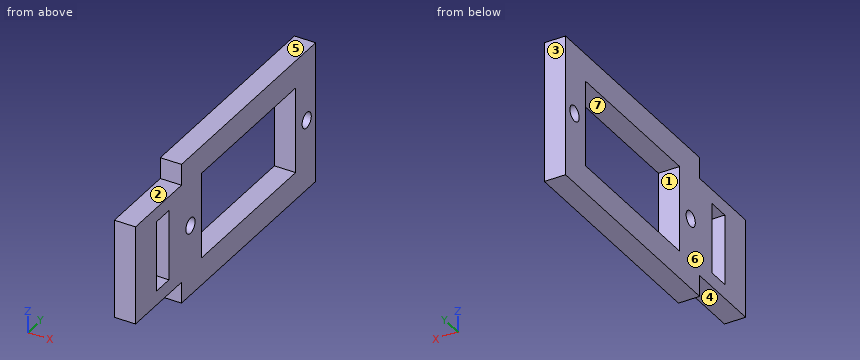
```python
from build123d import *

# Parameters (mm, degrees)
SKETCH1_W           = 20
SKETCH1_H           = 43.1
SKETCH1_W_2         = 10
SKETCH1_H_2         = 3
BOSS_EXTRUDE1_DEPTH = 3
SKETCH2_R           = 1.1
SKETCH2_W           = 12.2
SKETCH2_H           = 22.5
SKETCH2_W_2         = 3
SKETCH2_H_2         = 11
CUT_EXTRUDE1_DEPTH  = 3


with BuildPart() as part:
    # Sketch1 → Boss-Extrude1 (new body)
    with BuildSketch(Plane(origin=(0, 0, 0), x_dir=(0, 0, -1), z_dir=(1, 0, 0))):
        with Locations((10, 21.55)):
            Rectangle(SKETCH1_W, SKETCH1_H)
        with Locations((10, 6.5)):
            Rectangle(SKETCH1_W_2, SKETCH1_H_2, mode=Mode.SUBTRACT)
    extrude(amount=BOSS_EXTRUDE1_DEPTH)

    # Sketch2 → Cut-Extrude1 (cut)
    with BuildSketch(Plane.ZY):
        with Locations((-10, 40.95)):
            Circle(SKETCH2_R)
        with Locations((-10, 13.15)):
            Circle(SKETCH2_R)
        with Locations((-10, 27.05)):
            Rectangle(SKETCH2_W, SKETCH2_H)
        with Locations((-18.5, 5.5)):
            Rectangle(SKETCH2_W_2, SKETCH2_H_2)
        with Locations((-1.5, 5.5)):
            Rectangle(SKETCH2_W_2, SKETCH2_H_2)
    extrude(amount=-CUT_EXTRUDE1_DEPTH, mode=Mode.SUBTRACT)


solid = part.part
```
Model file for the job. Use its own axes, mm. Face numbers are marked on the shaded views. A direction names the side the tool comes from. Coordinates: 2 decimals unless noted, no trailing zeros. Write each loop counter-clockwise with the first axis right and the second up, starting at its lowest first coordinate (ties: lowest second). Pieces come first, ordered by that corner, then holes. Notation, with made-up numbers: (0, 69) - (32, 69) arc R25 ccw to (32, 96) - close; hole circle Ø1 at (-27.75, 89.25). An arc over 180 degrees is marked (long way). One line per item, written item: value. Start each with the question number.
1. Slice it at C-C (y = 13.15). Write the cut outline in (x, z).
2. Slice it at D-D (z = -12.75). Write the cut outline in (x, y), plus the area to 3 significant figures.
3. Probe line 1 (Y direction, x = 2.2, z = -10); line 2 (Y direction, x = 0.8, z = -14); line 3 (Z direction, x = 0.7, y = 30). List the from-to ranges inside material, lowest first. Write a range as from..to.
4. Mould opens along Z. For the marked faces 5, 6 and 7 say: released by +Z, released by -Z, zero draft, split by the parting line, or undercut.
5. Slice it at A-A (z = -10). Write the cut outline in (x, y).
6. Flat gauge pins, fed straight in: pin 1 (5 mm diameter, centred on y = 11, z = -12.5, fed in from -X); pin 2 (1.5 mm diameter, centred on x = 1.5, y = 7, fed in from -Z); pin 3 (1.3 mm diameter, centred on y = 13.15, z = -10, fed in from -X); pin 4 (1.5 mm diameter, centred on x = 2, y = 7, fed in from +Z). Where does each tip first touch, or does it go through?
7. Slice it at B-B (x = 1.4). Write the cut outline in (y, z).
8. Tool access for the marked faces 1, 2, 3 and 4: list every direction of +Z, -Z, +X, -X, +Y, -Y with a clear straight run to the whole face (end or side of a thin tool).
Answers below:
1. outline: (0, -20) - (3, -20) - (3, -11.1) - (0, -11.1) - close; (0, -8.9) - (3, -8.9) - (3, 0) - (0, 0) - close
2. outline: (0, 0) - (3, 0) - (3, 5) - (0, 5) - close; (0, 8) - (3, 8) - (3, 15.8) - (0, 15.8) - close; (0, 38.3) - (3, 38.3) - (3, 43.1) - (0, 43.1) - close
2. area: 52.8 mm^2
3. line 1: y = 0..5, 8..12.05, 14.25..15.8, 38.3..39.85, 42.05..43.1
3. line 2: y = 0..5, 8..15.8, 38.3..43.1
3. line 3: z = -20..-16.1, -3.9..0
4. face 5: released by +Z
4. face 6: zero draft
4. face 7: undercut
5. outline: (0, 0) - (3, 0) - (3, 5) - (0, 5) - close; (0, 8) - (3, 8) - (3, 12.05) - (0, 12.05) - close; (0, 14.25) - (3, 14.25) - (3, 15.8) - (0, 15.8) - close; (0, 38.3) - (3, 38.3) - (3, 39.85) - (0, 39.85) - close; (0, 42.05) - (3, 42.05) - (3, 43.1) - (0, 43.1) - close
6. pin 1: stops at x = 0
6. pin 2: stops at z = -17
6. pin 3: passes through
6. pin 4: stops at z = -3
7. outline: (0, -17) - (11, -17) - (11, -20) - (43.1, -20) - (43.1, 0) - (11, 0) - (11, -3) - (0, -3) - close; hole (5, -15) - (8, -15) - (8, -5) - (5, -5) - close; hole circle Ø2.2 at (13.15, -10); hole (15.8, -16.1) - (38.3, -16.1) - (38.3, -3.9) - (15.8, -3.9) - close; hole circle Ø2.2 at (40.95, -10)
8. face 1: +X, -X
8. face 2: +Z, +X, -X, -Y
8. face 3: +Z, -Z, +X, -X, +Y
8. face 4: -Z, +X, -X, -Y
